The drawing under review shows one solid part. Ordinate dimensions are in mm from its lowest x, y, z. A direction names the side the tool comes from. Coordinates: 2 decimals unless noted, no trailing zeros. Write each loop counter-clockwise with the first axis right and the second up, starting at its lowest first coordinate (ties: lowest second). Pieces come first, ordered by that corner, then holes.
1) We need section B-B on z = 8.5. Write out the cut boundary in (x, y).
2) We need section C-C on y = 12.5. Write out the cut boundary in (x, z).
3) Mouldability with a two-part tool opening along Y and no side actions: class the marked faces 4, 5 and 6 as pulls with the +Y half, pulls with the -Y half, needs draft (parallel to the pull), parting line crosses it, or undercut.
4) For the marked faces 1, 2 and 3, list the 3-axis set-ups (+Z, -Z, +X, -X, +Y, -Y) from which the entire face can be reached by the end or side of a thin tool; tool diameter is ignored.
5) We need section D-D on z = 47.5. Write out the cut boundary in (x, y).
6) We need section A-A on x = 8. Write out the cut boundary in (y, z).
7) Insertion check: P1, Ø5, axis at x = 7, z = 16, coming from the -Y side; P2, Ø3, axis at y = 19.5, z = 26.5, coming from the +X side; P3, Ø1.7, axis at y = 28, z = 13.5, coming from the +X side. Each pin has a flat end and moves straight along its axis. Give the tip position at first contact, or say it passes through.
8) To check wall thickness, follow line 1 along Y through (x, z) = (5.25, 44.5); line 2 along Y through (x, z) = (7, 51.5); line 3 along X through (y, z) = (19.5, 37.5). State the ranges of each line that lie inside material, in increasing order.
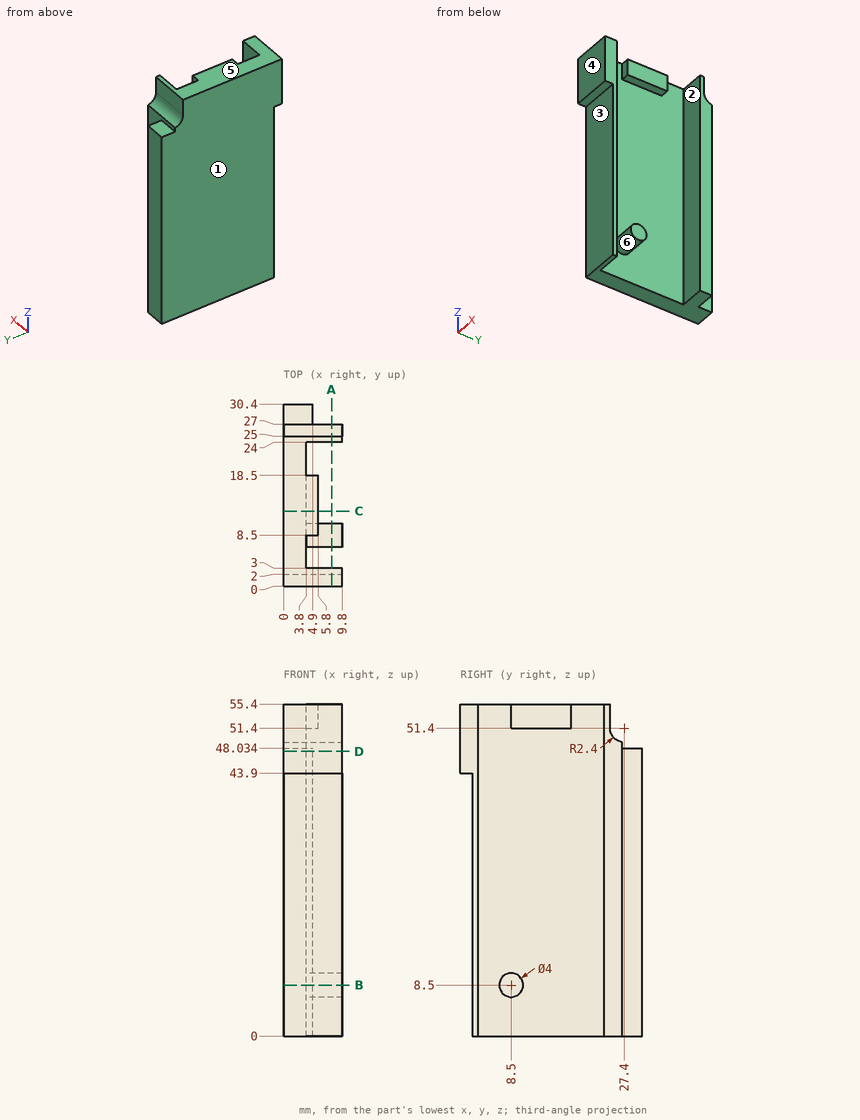
Result:
1. outline: (0, 2) - (9.8, 2) - (9.8, 3) - (3.8, 3) - (3.8, 6.5) - (9.8, 6.5) - (9.8, 10.5) - (3.8, 10.5) - (3.8, 24) - (9.8, 24) - (9.8, 27) - (4.9, 27) - (4.9, 30.4) - (0, 30.4) - close
2. outline: (0, 0) - (3.8, 0) - (3.8, 51.4) - (5.8, 51.4) - (5.8, 55.4) - (0, 55.4) - close
3. face 4: pulls with the -Y half
3. face 5: needs draft
3. face 6: undercut
4. face 1: +Z, -Z, -X, +Y, -Y
4. face 2: +Z, -Z, +X
4. face 3: -Z, +X, -X, -Y
5. outline: (0, 0) - (9.8, 0) - (9.8, 3) - (3.8, 3) - (3.8, 24) - (9.8, 24) - (9.8, 27) - (4.9, 27) - (4.9, 30.4) - (0, 30.4) - close
6. outline: (0, 43.9) - (2, 43.9) - (2, 0) - (3, 0) - (3, 55.4) - (0, 55.4) - close; circle Ø4 at (8.5, 8.5); (24, 0) - (27, 0) - (27, 49.03) arc R2.4 cw to (25, 51.4) - (25, 55.4) - (24, 55.4) - close
7. P1: stops at y = 2
7. P2: stops at x = 3.8
7. P3: stops at x = 4.9
8. line 1: y = 0 to 3, 24 to 27
8. line 2: y = 0 to 3, 24 to 25
8. line 3: x = 0 to 3.8
